Geometry: final body of the model. Coordinates: model frame, mm. Face numbers are marked on the shaded views. A direction names the side the tool comes from. Give positions to 0.01 mm unless a question says otherwise; leave off trailing zeros. Loops run counter-clockwise (first coordinate to the right, second up) from the corner with the lowest first, then second, coordinate; pieces in that order, holes last. Notation, with made-up numbers: (-30.5, 79.25) - (-15.5, 79.25) arc R4 ccw to (-15.5, 86.25) - close; hole circle Ø7 at (77.5, 80). An arc over 180 degrees is marked (long way). Answer in a Markdown table with one row per item.
from build123d import *

# Parameters (mm, degrees)
F0_R       = 30
F1_DEPTH   = 13
F3_DEPTH   = 25
F5_DEPTH   = 25
F7_DEPTH   = 25
F9_DEPTH   = 25
F10_R      = 10
F10_R_2    = 7
F11_DEPTH  = 10
F11_FACE_R = 7
F12_DEPTH  = 39.351137
F13_R      = 3
F14_R      = 3


with BuildPart() as f1:
    # F0 (on Top) → F1 (new body)
    with BuildSketch(Plane.XY):
        Circle(F0_R)
    extrude(amount=F1_DEPTH)

    # F2 (on face) → F3 (cut)
    with BuildSketch(Plane.XY.offset(13)):
        with BuildLine():
            Line((5, -29.580399), (5, -20))
            ThreePointArc((5, -20), (0, -25), (-5, -20))
            Line((-5, -20), (-5, -29.580399))
            ThreePointArc((-5, -29.580399), (0, -30), (5, -29.580399))
        make_face()
        with BuildLine():
            ThreePointArc((-5, -20), (0, -25), (5, -20))
            ThreePointArc((5, -20), (0, -15), (-5, -20))
        make_face()
    extrude(amount=-F3_DEPTH, mode=Mode.SUBTRACT)

    # F4 (on face) → F5 (cut)
    with BuildSketch(Plane.XY.offset(13)):
        with BuildLine():
            ThreePointArc((-5, 20), (0, 15), (5, 20))
            ThreePointArc((5, 20), (0, 25), (-5, 20))
        make_face()
        with BuildLine():
            ThreePointArc((-5, 20), (0, 25), (5, 20))
            Line((5, 20), (5, 29.580399))
            ThreePointArc((5, 29.580399), (0, 30), (-5, 29.580399))
            Line((-5, 29.580399), (-5, 20))
        make_face()
    extrude(amount=-F5_DEPTH, mode=Mode.SUBTRACT)

    # F6 (on face) → F7 (join)
    with BuildSketch(Plane.XY.offset(13)):
        with BuildLine():
            ThreePointArc((0, -13.5), (9.545942, -9.545942), (13.5, 0))
            ThreePointArc((13.5, 0), (9.545942, 9.545942), (0, 13.5))
            ThreePointArc((0, 13.5), (-13.5, 0), (0, -13.5))
        make_face()
        with BuildLine():
            ThreePointArc((0, 13.5), (9.545942, 9.545942), (13.5, 0))
            ThreePointArc((13.5, 0), (9.545942, -9.545942), (0, -13.5))
            Line((0, -13.5), (17, -13.5))
            Line((17, -13.5), (17, 13.5))
            Line((17, 13.5), (0, 13.5))
        make_face()
    extrude(amount=F7_DEPTH)

    # F8 (on Front) → F9 (cut, symmetric)
    with BuildSketch(Plane.XZ):
        Polygon((-14.918525, 36.73033), (17, 18.302161), (17, 39.234225), (-14.918525, 39.234225), align=None)
    extrude(amount=F9_DEPTH, both=True, mode=Mode.SUBTRACT)

    # F10 (on face) → F11 (cut)
    with BuildSketch(Plane(origin=(12.175068, 0, 21.087837), x_dir=(0.866025, 0, -0.5), z_dir=(0.5, 0, 0.866025))):
        with Locations((-14.058558, 0)):
            Circle(F10_R)
        with Locations((-14.058558, 0)):
            Circle(F10_R_2, mode=Mode.SUBTRACT)
    extrude(amount=-F11_DEPTH, mode=Mode.SUBTRACT)

    # F11_face (on face) → F12 (cut, through all)
    with BuildSketch(Plane(origin=(0, 0, 28.117116), x_dir=(0, 1, 0), z_dir=(0.5, 0, 0.866025))):
        Circle(F11_FACE_R)
    extrude(amount=-F12_DEPTH, mode=Mode.SUBTRACT)

    # F13
    f13_edges = [f1.edges().sort_by_distance(p)[0] for p in [
        (-30, 0, 13),
    ]]
    fillet(f13_edges, radius=F13_R)

    # F14
    f14_edges = [f1.edges().sort_by_distance(p)[0] for p in [
        (30, 0, 13),
    ]]
    fillet(f14_edges, radius=F14_R)


solid = f1.part
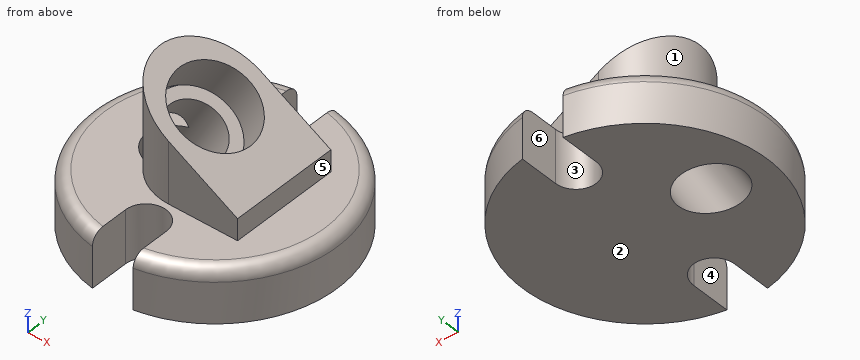
Q1. Cut plane A-A (y = 0). Output: boundary loops of the cut face in (x, z).
Check values:
| item | result |
|---|---|
| outline | (-30, 0) - (-24.32, 0) - (-16.81, 13) - (-27, 13) arc R3 ccw to (-30, 10) - close; (-13.5, 18.73) - (-11.06, 22.96) - (-13.5, 24.36) - close; (-13.5, 24.73) - (-8.66, 33.12) - (-13.5, 35.91) - close; (-8.15, 0) - (30, 0) - (30, 10) arc R3 ccw to (27, 13) - (17, 13) - (17, 18.3) - (8.66, 23.12) - (3.66, 14.46) - (1.06, 15.96) - close |
Q2. Material intervals for line 1 along Z through (x, y) = (9.5, 17.5); line 2 along X through (y, z) = (-18.5, 11); line 3 along Y through (x, z) = (8, 15.5), sorted ascending.
Check values:
| item | result |
|---|---|
| line 1 | 0 to 13 |
| line 2 | -23.4 to -4.77, 4.77 to 23.4 |
| line 3 | -13.5 to 13.5 |
Q3. Draft query along X for the marked faces 1, 2 and 3. Return one class per face: pulls with the +X half, pulls with the -X half, needs draft (parallel to the pull), parting line crosses it, or undercut.
Check values:
| item | result |
|---|---|
| face 1 | pulls with the -X half |
| face 2 | needs draft |
| face 3 | undercut |
Q4. Reachability of the marked faces 4, 5 and 6 from +Z, -Z, +X, -X, +Y, -Y: full face, straight path, thin tool, end or side. Return the list, or none.
Check values:
| item | result |
|---|---|
| face 4 | +Z, -Z, -Y |
| face 5 | +Z, +X, +Y, -Y |
| face 6 | +Z, -Z, +Y |
Q5. First-contact query: pin 1 (1 mm diameter, centred on x = -4.5, y = 19, fed in from +Z); pin 2 (3 mm diameter, centred on y = -26, z = 7.5, fed in from -X); pin 3 (3 mm diameter, centred on x = -11.5, z = 21.5, fed in from -Y). Flat tips, straight axial feed; report the tip coordinate or a pass-through.
Check values:
| item | result |
|---|---|
| pin 1 | z = 13 |
| pin 2 | x = -17.31 |
| pin 3 | y = -9.07 |
